from build123d import *

# Parameters (mm, degrees)
MODEL_R             = 1.5
MODEL_R_2           = 8.25
BOSS_EXTRUDE1_DEPTH = 2


with BuildPart() as part:
    # Model → Boss-Extrude1 (new body)
    with BuildSketch(Plane.XY):
        with BuildLine():
            Line((-21.5, 30), (21.5, 30))
            ThreePointArc((21.5, 30), (23.267766953, 29.267766953), (24, 27.5))
            Line((24, 27.5), (24, 2.5))
            ThreePointArc((24, 2.5), (23.267766953, 0.732233047), (21.5, 0))
            Line((21.5, 0), (-21.5, 0))
            ThreePointArc((-21.5, 0), (-23.267766953, 0.732233047), (-24, 2.5))
            Line((-24, 2.5), (-24, 27.5))
            ThreePointArc((-24, 27.5), (-23.267766953, 29.267766953), (-21.5, 30))
        make_face()
        with Locations((18, 15)):
            Circle(MODEL_R, mode=Mode.SUBTRACT)
        with Locations(Location((-18, 15, 0), (0, 0, 180))):
            Circle(MODEL_R, mode=Mode.SUBTRACT)
        with Locations((0, 15)):
            Circle(MODEL_R_2, mode=Mode.SUBTRACT)
    extrude(amount=BOSS_EXTRUDE1_DEPTH)


solid = part.part
Could you check a few things on this model? Use its own coordinates, in mm. Coordinates: 2 decimals unless noted, no trailing zeros. Loops run counter-clockwise (first coordinate to the right, second up) from the corner with the lowest first, then second, coordinate; pieces in that order, holes last. Notation, with made-up numbers: (40.5, -2) -> (66.5, -2) arc R14 cw to (66.5, 13) -> close; hole circle Ø5 at (1.25, -18). An arc over 180 degrees is marked (long way). Answer in a Markdown table with one row per item.
(1) Will this pin go through, and if not, where does the flat tip stop? pin 1 Ø2 at (x, y) = (-11.5, 7) entering from -Z.
Results found:
| item | result |
|---|---|
| pin 1 | stops at z = 0 |
(2) Imagine slicing it at C-C (z = 1.1). List the corners of the cut face in (x, y) for me, plus the area to 3 significant figures.
Results found:
| item | result |
|---|---|
| outline | (-24, 2.5) arc R2.5 ccw to (-21.5, 0) -> (21.5, 0) arc R2.5 ccw to (24, 2.5) -> (24, 27.5) arc R2.5 ccw to (21.5, 30) -> (-21.5, 30) arc R2.5 ccw to (-24, 27.5) -> close; hole circle Ø3 at (-18, 15); hole circle Ø16.5 at (0, 15); hole circle Ø3 at (18, 15) |
| area | 1,210 mm^2 |
(3) Imagine slicing it at B-B (y = 12.25). List the corners of the cut face in (x, z) for me.
Results found:
| item | result |
|---|---|
| outline | (-24, 0) -> (-7.78, 0) -> (-7.78, 2) -> (-24, 2) -> close; (7.78, 0) -> (24, 0) -> (24, 2) -> (7.78, 2) -> close |
(4) If I drill on probe 1 along Y at (x, z) = (0, 1.35); probe 2 along Y at (x, z) = (18, 1.6); probe 3 along X at (y, z) = (19.5, 0.35), over which ranges is the centre line in solid material (lowest first)?
Results found:
| item | result |
|---|---|
| probe 1 | y = 0 to 6.75, 23.25 to 30 |
| probe 2 | y = 0 to 13.5, 16.5 to 30 |
| probe 3 | x = -24 to -6.91, 6.91 to 24 |
(5) Thinking about a two-plate mould opening in X: for faces 1 (the face through (16.5, 15.07, 0.99)), 2 (the face through (0, 30, 1)), 3 (the face through (-23.248, 0.713, 0.986)), which applies, released by +X, released by -X, zero draft, split by the parting line, or undercut?
Results found:
| item | result |
|---|---|
| face 1 | undercut |
| face 2 | zero draft |
| face 3 | released by -X |
(6) Imagine slicing it at A-A (x = -18). List the corners of the cut face in (y, z) for me, plus the area to 3 significant figures.
Results found:
| item | result |
|---|---|
| outline | (0, 0) -> (13.5, 0) -> (13.5, 2) -> (0, 2) -> close; (16.5, 0) -> (30, 0) -> (30, 2) -> (16.5, 2) -> close |
| area | 54.0 mm^2 |
